Check sheet for the modelled part. Datum: model origin and axes. Units: mm. Face numbers are marked on the shaded views. A direction names the side the tool comes from. Give positions to 0.01 mm unless a question says otherwise; leave off trailing zeros. Loops run counter-clockwise (first coordinate to the right, second up) from the corner with the lowest first, then second, coordinate; pieces in that order, holes last. Notation, with made-up numbers: M 14.5,46.25 L 29.5,46.25 A6 ccw 29.5,50.25 Z; hole C 55.25,75 d8. An arc over 180 degrees is marked long. One line per question, with ' | ' between items. Start each with the question number.
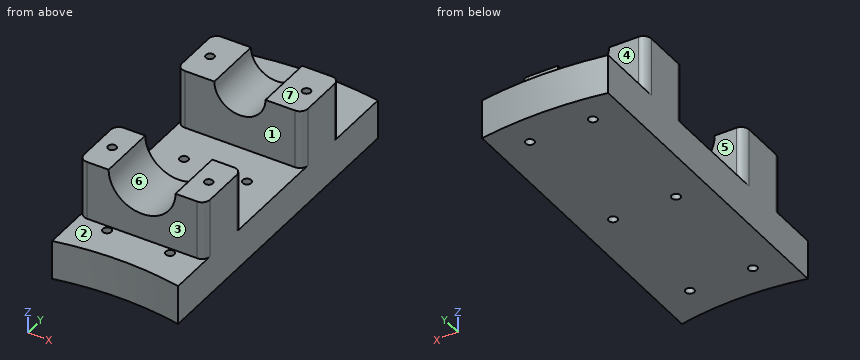
from build123d import *

# Parameters (mm, degrees)
SKETCH1_R               = 1.1
BOSS_EXTRUDE7_DEPTH     = 10
CUT_EXTRUDE4_DEPTH      = 74.565999455
CUT_EXTRUDE4_DEPTH_BACK = 74.565999455
SKETCH1_9_R             = 1.1
SKETCH6_W               = 32
SKETCH6_H               = 15
BOSS_EXTRUDE8_DEPTH     = 30
CUT_EXTRUDE5_DEPTH      = 16
CUT_EXTRUDE6_DEPTH      = 22
SKETCH10_R              = 1.05
CUT_EXTRUDE7_DEPTH      = 10
FILLET1_R               = 2


with BuildPart() as part:
    # Sketch1 → Boss-Extrude7 (new body)
    with BuildSketch(Plane.XY):
        with BuildLine():
            Line((-2.62989834, -18.895475724), (-2.62989834, 62.787818526))
            ThreePointArc((-2.62989834, 62.787818526), (-18.62989834, 64.130541996), (-34.62989834, 62.787818526))
            Line((-34.62989834, 62.787818526), (-34.62989834, -18.895475724))
            ThreePointArc((-34.62989834, -18.895475724), (-18.62989834, -17.279147493), (-2.62989834, -18.895475724))
        make_face()
        with Locations((-26.62989834, -9.279147493)):
            Circle(SKETCH1_R, mode=Mode.SUBTRACT)
        with Locations((-10.62989834, -9.279147493)):
            Circle(SKETCH1_R, mode=Mode.SUBTRACT)
    extrude(amount=BOSS_EXTRUDE7_DEPTH)

    # Sketch1_9 → Cut-Extrude4 (cut, two sides: drawn at the far end of the back side and taken through both)
    with BuildSketch(Plane.XY.offset(-CUT_EXTRUDE4_DEPTH_BACK)):
        with Locations((-10.62989834, 56.130541996)):
            Circle(SKETCH1_9_R)
        with Locations(Location((-26.62989834, 56.130541996, 0), (0, 0, 180))):
            Circle(SKETCH1_9_R)
        with Locations((-10.62989834, 22.130541996)):
            Circle(SKETCH1_9_R)
        with Locations(Location((-26.62989834, 22.130541996, 0), (0, 0, 180))):
            Circle(SKETCH1_9_R)
    extrude(amount=CUT_EXTRUDE4_DEPTH + CUT_EXTRUDE4_DEPTH_BACK, mode=Mode.SUBTRACT)

    # Sketch6 → Boss-Extrude8 (add)
    with BuildSketch(Plane.XY.offset(10)):
        with Locations((-18.62989834, -0.369458004)):
            Rectangle(SKETCH6_W, SKETCH6_H)
        with Locations((-18.62989834, 39.630541996)):
            Rectangle(SKETCH6_W, SKETCH6_H)
    extrude(amount=BOSS_EXTRUDE8_DEPTH)

    # Sketch7 → Cut-Extrude5 (cut)
    with BuildSketch(Plane(origin=(0, 47.130541996, 0), x_dir=(1, 0, 0), z_dir=(0, 1, 0))):
        with BuildLine():
            Line((-2.62989834, -40), (-2.62989834, -25))
            Line((-2.62989834, -25), (-12.12989834, -25))
            ThreePointArc((-12.12989834, -25), (-18.62989834, -18.5), (-25.12989834, -25))
            Line((-25.12989834, -25), (-34.62989834, -25))
            Line((-34.62989834, -25), (-34.62989834, -40))
            Line((-34.62989834, -40), (-2.62989834, -40))
        make_face()
    extrude(amount=-CUT_EXTRUDE5_DEPTH, mode=Mode.SUBTRACT)

    # Sketch8 → Cut-Extrude6 (cut)
    with BuildSketch(Plane(origin=(0, 7.130541996, 0), x_dir=(1, 0, 0), z_dir=(0, 1, 0))):
        with BuildLine():
            Line((-2.62989834, -25), (-10.12989834, -25))
            ThreePointArc((-10.12989834, -25), (-18.62989834, -16.5), (-27.12989834, -25))
            Line((-27.12989834, -25), (-34.62989834, -25))
            Line((-34.62989834, -25), (-34.62989834, -40))
            Line((-34.62989834, -40), (-2.62989834, -40))
            Line((-2.62989834, -40), (-2.62989834, -25))
        make_face()
    extrude(amount=-CUT_EXTRUDE6_DEPTH, mode=Mode.SUBTRACT)

    # Sketch10 → Cut-Extrude7 (cut)
    with BuildSketch(Plane.XY.offset(25)):
        with Locations((-30.87989834, -0.369458004)):
            Circle(SKETCH10_R)
        with Locations(Location((-30.87989834, 39.630541996, 0), (0, 0, 180))):
            Circle(SKETCH10_R)
        with Locations(Location((-6.37989834, -0.369458004, 0), (0, 0, 180))):
            Circle(SKETCH10_R)
        with Locations((-6.37989834, 39.630541996)):
            Circle(SKETCH10_R)
    extrude(amount=-CUT_EXTRUDE7_DEPTH, mode=Mode.SUBTRACT)

    # Fillet1
    fillet1_edges = [part.edges().sort_by_distance(p)[0] for p in [
        (-34.62989834, 7.130541996, 17.5),
        (-2.62989834, 7.130541996, 17.5),
        (-2.62989834, -7.869458004, 17.5),
        (-34.62989834, -7.869458004, 17.5),
        (-2.62989834, 32.130541996, 17.5),
        (-34.62989834, 32.130541996, 17.5),
        (-34.62989834, 47.130541996, 17.5),
        (-2.62989834, 47.130541996, 17.5),
    ]]
    fillet(fillet1_edges, radius=FILLET1_R)


solid = part.part
Q1. Access from +Z, -Z, +X, -X, +Y, -Y to the whole of each face (thin tool, end or side, straight path). Record for the marked faces 4, 5, 6 and 7.
Q2. Draft check along Y on the marked faces 1, 2 and 3. Enter one of: released by +Y, released by -Y, zero draft, split by the parting line, or undercut.
Q3. Cross-section at C-C (z = 4). Record the cut outline in (x, y).
Q4. Depth check by flat-ended pin: P1, Ø5, axis at x = -6, z = 14.5, coming from the +Y side; P2, Ø1.3, axis at x = -10.63, y = 22.13, coming from the +Z side; P3, Ø12, axis at x = -23.5, z = 16.5, coming from the -Y side; P4, Ø2.5, axis at x = -6, y = 0, coming from the +Z side. Enter the tip coordinate at first touch or a pass-through.
Q5. Cross-section at B-B (x = -15). Record the cut outline in (y, z), and give its area (3 significant figures).
Q6. Cross-section at A-A (y = -3). Record the cut outline in (x, z), and give its area (3 significant figures).
Q7. Material ranges on probe 1 along Y at (x, z) = (-10.5, 12.75); probe 2 along X at (y, z) = (39, 23); probe 3 along Z at (x, y) = (-20.5, 58), recorded low to high. Write a range as from..to.
Q8. Cross-section at D-D (y = 35). Record the cut outline in (x, z).
Solved:
1) face 4: +Z, +X, -X, +Y | face 5: +Z, +X, -X | face 6: +Z, -Y | face 7: +Z, +X, -X, +Y, -Y
2) face 1: undercut | face 2: zero draft | face 3: released by -Y
3) outline: M -34.63,-18.9 A80 cw -2.63,-18.9 L -2.63,62.79 A96 ccw -34.63,62.79 Z; hole C -26.63,-9.28 d2.2; hole C -26.63,22.13 d2.2; hole C -26.63,56.13 d2.2; hole C -10.63,-9.28 d2.2; hole C -10.63,22.13 d2.2; hole C -10.63,56.13 d2.2
4) P1: stops at y = 47.13 | P2: passes through | P3: stops at y = -7.87 | P4: stops at z = 25
5) outline: M -17.36,0 L 64.06,0 L 64.06,10 L 47.13,10 L 47.13,19.61 L 32.13,19.61 L 32.13,10 L 7.13,10 L 7.13,17.31 L -7.87,17.31 L -7.87,10 L -17.36,10 Z | area: 1,070 mm²
6) outline: M -34.63,0 L -2.63,0 L -2.63,25 L -10.13,25 A8.5 cw -27.13,25 L -34.63,25 Z | area: 687 mm²
7) probe 1: y = -7.87..7.13, 32.13..47.13 | probe 2: x = -34.63..-31.72, -30.04..-24.81, -12.45..-7.22, -5.54..-2.63 | probe 3: z = 0..10
8) outline: M -34.63,0 L -2.63,0 L -2.63,25 L -12.13,25 A6.5 cw -25.13,25 L -34.63,25 Z
